Job drawing, mm, ordinate dimensions from the low corner. One solid piece. Give positions to 0.01 mm unless a question says otherwise; leave off trailing zeros. Loops run counter-clockwise (first coordinate to the right, second up) from the corner with the lowest first, then second, coordinate; pieces in that order, holes last.
Item 1: Mould opens along Z. For the marked faces 1, 2 and 3 say: released by +Z, released by -Z, zero draft, split by the parting line, or undercut.
Item 2: Probe probe 1 along Z at (x, y) = (3.45, 2.6); probe 2 along Z at (x, y) = (2, 3.35) (1 decimal); probe 3 along X at (y, z) = (4.2, 4). List the from-to ranges inside material, lowest first.
Item 3: Saw through at B-B on z = 5. Give the cut face in (x, y).
Item 4: Saw through at A-A on x = 3.45. Give the cut face in (y, z).
Item 5: Saw through at D-D on x = 6.75. Give the cut face in (y, z).
Item 6: Saw through at C-C on y = 3. Give the cut face in (x, z).
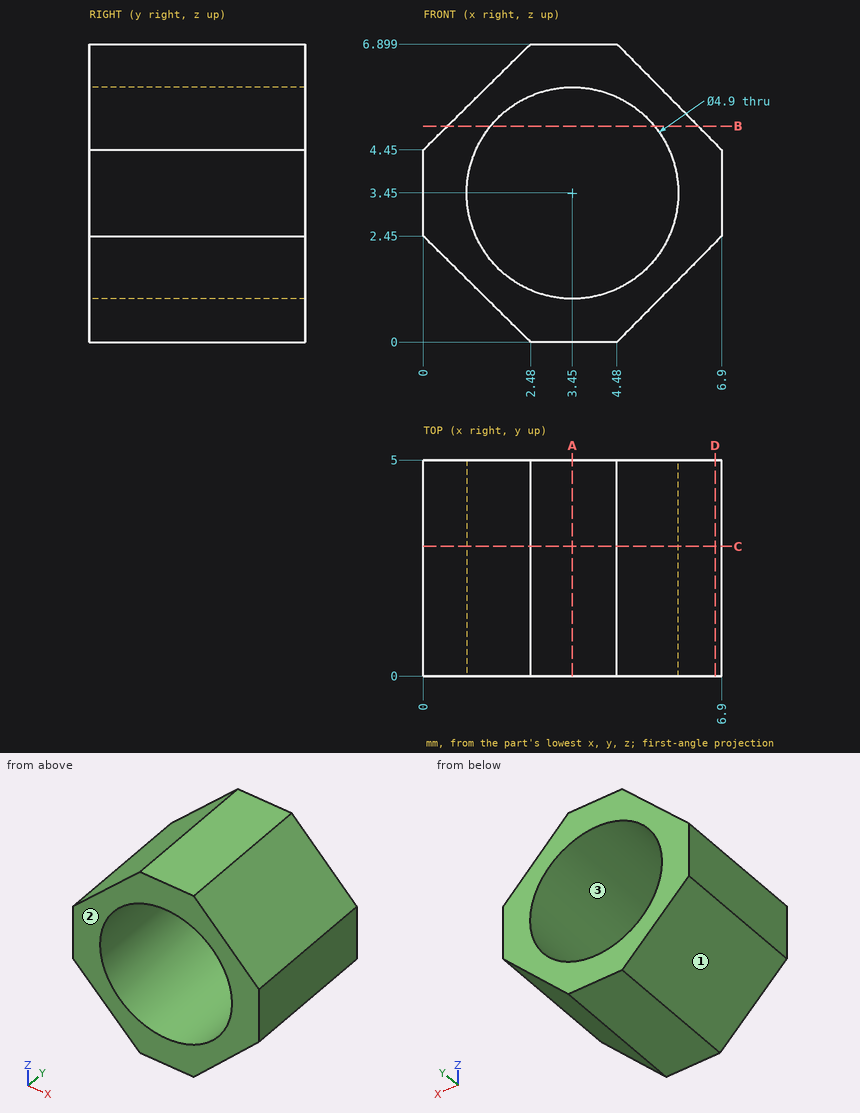
Results below:
1. face 1: released by -Z
1. face 2: zero draft
1. face 3: undercut
2. probe 1: z = 0 to 1, 5.9 to 6.9
2. probe 2: z = 0.5 to 1.5, 5.4 to 6.4
2. probe 3: x = 0 to 1.06, 5.84 to 6.9
3. outline: (0.56, 0) - (1.55, 0) - (1.55, 5) - (0.56, 5) - close; (5.35, 0) - (6.36, 0) - (6.36, 5) - (5.35, 5) - close
4. outline: (0, 0) - (5, 0) - (5, 1) - (0, 1) - close; (0, 5.9) - (5, 5.9) - (5, 6.9) - (0, 6.9) - close
5. outline: (0, 2.3) - (5, 2.3) - (5, 4.6) - (0, 4.6) - close
6. outline: (0, 2.45) - (2.48, 0) - (4.48, 0) - (6.9, 2.45) - (6.9, 4.45) - (4.48, 6.9) - (2.48, 6.9) - (0, 4.45) - close; hole circle Ø4.9 at (3.45, 3.45)
